from build123d import *

# Parameters (mm, degrees)
SKETCH1_R           = 1
BOSS_EXTRUDE1_DEPTH = 1
SKETCH2_R           = 2.4
BOSS_EXTRUDE2_DEPTH = 2.8


with BuildPart() as part:
    # Sketch1 → Boss-Extrude1 (new body)
    with BuildSketch(Plane.XY):
        with BuildLine():
            Line((-15.5, 7.5), (15.5, 7.5))
            ThreePointArc((15.5, 7.5), (16.207106781, 7.207106781), (16.5, 6.5))
            Line((16.5, 6.5), (16.5, -6.5))
            ThreePointArc((16.5, -6.5), (16.207106781, -7.207106781), (15.5, -7.5))
            Line((15.5, -7.5), (-15.5, -7.5))
            ThreePointArc((-15.5, -7.5), (-16.207106781, -7.207106781), (-16.5, -6.5))
            Line((-16.5, -6.5), (-16.5, 6.5))
            ThreePointArc((-16.5, 6.5), (-16.207106781, 7.207106781), (-15.5, 7.5))
        make_face()
        with Locations((-13.9, 0)):
            Circle(SKETCH1_R, mode=Mode.SUBTRACT)
        with Locations((13.6, 0)):
            Circle(SKETCH1_R, mode=Mode.SUBTRACT)
    extrude(amount=BOSS_EXTRUDE1_DEPTH)

    # Sketch2 → Boss-Extrude2 (add)
    with BuildSketch(Plane.XY.offset(1)):
        with Locations((-5.39, 0)):
            Circle(SKETCH2_R)
    extrude(amount=BOSS_EXTRUDE2_DEPTH)


solid = part.part
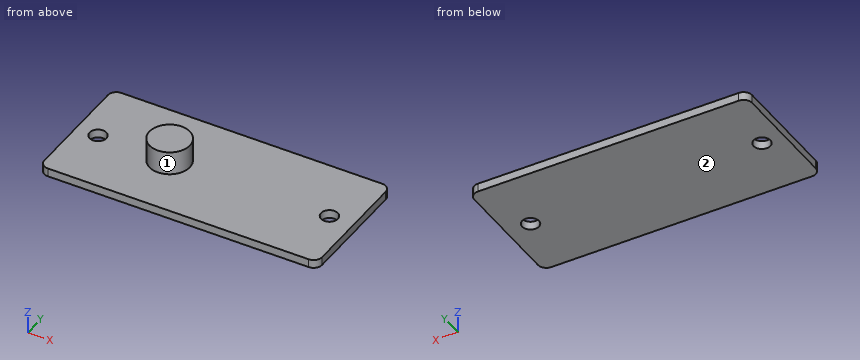
Verification items for the finished model (mm, model axes). Face numbers are marked on the shaded views. A direction names the side the tool comes from. Give positions to 0.01 mm unless a question says otherwise; leave off trailing zeros. Order: outer loops, then holes, each group sorted by start corner. A loop starts at its lowest first (then second) coordinate and runs counter-clockwise, first axis right, second up. Notation, with made-up numbers: (-11, 42.25) -> (14, 42.25) arc R30 ccw to (14, 72.25) -> close; hole circle Ø9 at (72.25, 4.5). An arc over 180 degrees is marked (long way). Answer as CSV lines item,"result".
Q1. Depth check by flat-ended pin: pin 1 (1 mm diameter, centred on x = 12.5, y = 2, fed in from +Z); pin 2 (1.6 mm diameter, centred on x = -13.9, y = 0, fed in from -Z) (3 decimals). Enter the tip coordinate at first touch or a pass-through.
Solutions:
pin 1,"stops at z = 1"
pin 2,"passes through"
Q2. Scan lines: probe 1 along Y at (x, z) = (-13.9, 0.2); probe 2 along Z at (x, y) = (15.5, 3.5); probe 3 along Y at (x, z) = (-5, 2.6). Record each from-to range of solid material in increasing order.
Solutions:
probe 1,"y = -7.5 to -1, 1 to 7.5"
probe 2,"z = 0 to 1"
probe 3,"y = -2.37 to 2.37"
Q3. Access from +Z, -Z, +X, -X, +Y, -Y to the whole of each face (thin tool, end or side, straight path). Record for the marked faces 1 and 2.
Solutions:
face 1,"+Z"
face 2,"-Z, +X, -X, +Y, -Y"
Q4. Sectioned sample at A-A on x = -13.9. Record the cut outline in (y, z).
Solutions:
outline,"(-7.5, 0) -> (-1, 0) -> (-1, 1) -> (-7.5, 1) -> close; (1, 0) -> (7.5, 0) -> (7.5, 1) -> (1, 1) -> close"
Q5. Sectioned sample at B-B on y = 0. Record the cut outline in (x, z), plus the area to 3 significant figures.
Solutions:
outline,"(-16.5, 0) -> (-14.9, 0) -> (-14.9, 1) -> (-16.5, 1) -> close; (-12.9, 0) -> (12.6, 0) -> (12.6, 1) -> (-2.99, 1) -> (-2.99, 3.8) -> (-7.79, 3.8) -> (-7.79, 1) -> (-12.9, 1) -> close; (14.6, 0) -> (16.5, 0) -> (16.5, 1) -> (14.6, 1) -> close"
area,"42.4 mm²"
Q6. Sectioned sample at C-C on x = -5.39. Record the cut outline in (y, z).
Solutions:
outline,"(-7.5, 0) -> (7.5, 0) -> (7.5, 1) -> (2.4, 1) -> (2.4, 3.8) -> (-2.4, 3.8) -> (-2.4, 1) -> (-7.5, 1) -> close"
Q7. Sectioned sample at D-D on x = 13. Record the cut outline in (y, z).
Solutions:
outline,"(-7.5, 0) -> (-0.8, 0) -> (-0.8, 1) -> (-7.5, 1) -> close; (0.8, 0) -> (7.5, 0) -> (7.5, 1) -> (0.8, 1) -> close"
